Geometry: final body of the model. Coordinates: model frame, mm. Face numbers are marked on the shaded views. A direction names the side the tool comes from. Coordinates: 2 decimals unless noted, no trailing zeros. Write each loop counter-clockwise with the first axis right and the second up, starting at its lowest first coordinate (ties: lowest second). Pieces come first, ordered by that corner, then holes. Notation, with made-up numbers: (16.5, 84) - (45.5, 84) arc R24 cw to (45.5, 111) - close; hole circle Ø4 at (73.25, -14). An arc over 180 degrees is marked (long way). Put each result on its own line as item: value.
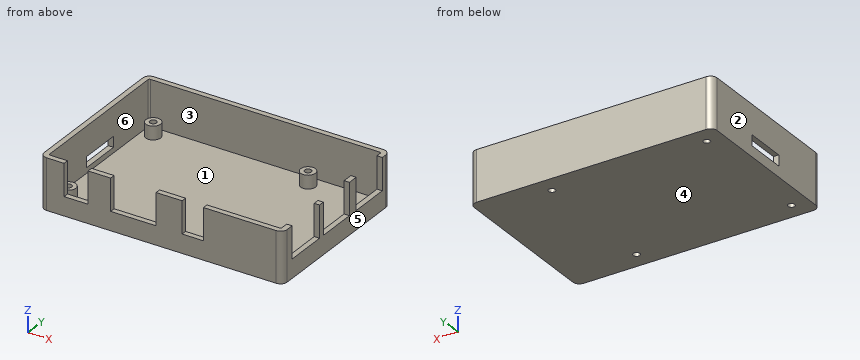
```python
from build123d import *

# Parameters (mm, degrees)
F0_W      = 87
F0_H      = 58
F1_DEPTH  = 2
F2_DEPTH  = 19
F3_R      = 2.75
F3_R_2    = 1.25
F4_DEPTH  = 5
F5_W      = 9
F5_H      = 2
F5_W_2    = 17
F5_W_3    = 8
F5_W_4    = 2
F5_H_2    = 15.9
F5_H_3    = 15.1
F6_DEPTH  = 12
F7_W      = 15.6
F7_H      = 4
F8_DEPTH  = 5
F9_R      = 0.5
F10_DEPTH = 2


with BuildPart() as f1:
    # F0 (on Top) → F1 (new body)
    with BuildSketch(Plane.XY):
        with BuildLine():
            ThreePointArc((0, 2.5), (0.732233047, 0.732233047), (2.5, 0))
            Line((2.5, 0), (88.5, 0))
            ThreePointArc((88.5, 0), (90.267766953, 0.732233047), (91, 2.5))
            Line((91, 2.5), (91, 59.5))
            ThreePointArc((91, 59.5), (90.267766953, 61.267766953), (88.5, 62))
            Line((88.5, 62), (2.5, 62))
            ThreePointArc((2.5, 62), (0.732233047, 61.267766953), (0, 59.5))
            Line((0, 59.5), (0, 2.5))
        make_face()
        with Locations((45.5, 31)):
            Rectangle(F0_W, F0_H, mode=Mode.SUBTRACT)
        with Locations((45.5, 31)):
            Rectangle(F0_W, F0_H)
    extrude(amount=F1_DEPTH)

    # F0 (on Top) → F2 (join)
    with BuildSketch(Plane.XY):
        with BuildLine():
            ThreePointArc((0, 2.5), (0.732233047, 0.732233047), (2.5, 0))
            Line((2.5, 0), (88.5, 0))
            ThreePointArc((88.5, 0), (90.267766953, 0.732233047), (91, 2.5))
            Line((91, 2.5), (91, 59.5))
            ThreePointArc((91, 59.5), (90.267766953, 61.267766953), (88.5, 62))
            Line((88.5, 62), (2.5, 62))
            ThreePointArc((2.5, 62), (0.732233047, 61.267766953), (0, 59.5))
            Line((0, 59.5), (0, 2.5))
        make_face()
        with Locations((45.5, 31)):
            Rectangle(F0_W, F0_H, mode=Mode.SUBTRACT)
    extrude(amount=F2_DEPTH)

    # F3 (on face) → F4 (join)
    with BuildSketch(Plane.XY.offset(2)):
        with Locations((6.5, 55.5)):
            Circle(F3_R)
        with Locations((6.5, 55.5)):
            Circle(F3_R_2, mode=Mode.SUBTRACT)
        with Locations((64.5, 6.5)):
            Circle(F3_R)
        with Locations((64.5, 6.5)):
            Circle(F3_R_2, mode=Mode.SUBTRACT)
        with Locations((6.5, 6.5)):
            Circle(F3_R)
        with Locations((6.5, 6.5)):
            Circle(F3_R_2, mode=Mode.SUBTRACT)
        with Locations((64.5, 55.5)):
            Circle(F3_R)
        with Locations((64.5, 55.5)):
            Circle(F3_R_2, mode=Mode.SUBTRACT)
    extrude(amount=F4_DEPTH)

    # F5 (on face) → F6 (cut)
    with BuildSketch(Plane.XY.offset(19)):
        with Locations((13.55, 1)):
            Rectangle(F5_W, F5_H)
        with Locations((35, 1)):
            Rectangle(F5_W_2, F5_H)
        with Locations((57.25, 1)):
            Rectangle(F5_W_3, F5_H)
        with Locations((90, 13.25)):
            Rectangle(F5_W_4, F5_H_2)
        with Locations((90, 30.95)):
            Rectangle(F5_W_4, F5_H_3)
        with Locations((90, 49.95)):
            Rectangle(F5_W_4, F5_H_3)
    extrude(amount=-F6_DEPTH, mode=Mode.SUBTRACT)

    # F7 (on face) → F8 (cut)
    with BuildSketch(Plane(origin=(0, 0, 0), x_dir=(0, -1, 0), z_dir=(-1, 0, 0))):
        with Locations((-31.7, 6)):
            Rectangle(F7_W, F7_H)
    extrude(amount=-F8_DEPTH, mode=Mode.SUBTRACT)

    # F9
    f9_edges = [f1.edges().sort_by_distance(p)[0] for p in [
        (2, 60, 10.5),
        (89, 60, 10.5),
        (2, 2, 10.5),
        (89, 2, 10.5),
    ]]
    fillet(f9_edges, radius=F9_R)

    # F10 (cut, through all): faces of the model
    f10_faces = [f1.faces().sort_by_distance(p)[0] for p in [
        (6.5, 55.5, 2),
        (64.5, 55.5, 2),
        (64.5, 6.5, 2),
        (6.5, 6.5, 2),
    ]]
    extrude(f10_faces, amount=-F10_DEPTH, mode=Mode.SUBTRACT)


solid = f1.part
```
1. Ray query, probe 1 along Y at (x, z) = (64.5, 1.6); probe 2 along X at (y, z) = (20, 6); probe 3 along Y at (x, z) = (48, 6.25). Return the intervals inside material, ascending. Write a range as from..to.
Answer below:
probe 1: y = 0..5.25, 7.75..54.25, 56.75..62
probe 2: x = 0..2, 89..91
probe 3: y = 0..2, 60..62
2. Section query C-C (x = 6.5). Return loops of the section in (y, z).
Answer below:
outline: (0, 0) - (5.25, 0) - (5.25, 7) - (3.75, 7) - (3.75, 2) - (2, 2) - (2, 19) - (0, 19) - close; (7.75, 0) - (54.25, 0) - (54.25, 7) - (52.75, 7) - (52.75, 2) - (9.25, 2) - (9.25, 7) - (7.75, 7) - close; (56.75, 0) - (62, 0) - (62, 19) - (60, 19) - (60, 2) - (58.25, 2) - (58.25, 7) - (56.75, 7) - close
3. Pin query (flat end, axial travel): pin 1 Ø1 at (x, z) = (90, 13.5) entering from +Y; pin 2 Ø8 at (x, y) = (61.5, 37.5) entering from +Z; pin 3 Ø2 at (x, y) = (64.5, 6.5) entering from +Z; pin 4 Ø0.6 at (y, z) = (0.5, 14.5) entering from -X. Return the tip coordinate at first contact, or that it passes through.
Answer below:
pin 1: stops at y = 61.79
pin 2: stops at z = 2
pin 3: passes through
pin 4: stops at x = 0.67
4. Section query A-A (z = 5). Count the separate pieces of the cut face and the enclosed holes in it, then the cut area to 3 significant figures.
Answer below:
separate pieces: 5
enclosed holes: 4
area: 635 mm²
5. Section query D-D (x = 71.5). Return loops of the section in (y, z).
Answer below:
outline: (0, 0) - (62, 0) - (62, 19) - (60, 19) - (60, 2) - (2, 2) - (2, 19) - (0, 19) - close
6. Mould query, pull axis X, two halves, no side actions, for the marked faces 1, 2, 3 and 4. Classes: +X half, -X half, draft (parallel to the pull), parting line (faces both ways), or undercut.
Answer below:
face 1: undercut
face 2: -X half
face 3: undercut
face 4: draft
7. Section query B-B (y = 55.5). Return loops of the section in (x, z).
Answer below:
outline: (0, 0) - (5.25, 0) - (5.25, 7) - (3.75, 7) - (3.75, 2) - (2, 2) - (2, 19) - (0, 19) - close; (7.75, 0) - (63.25, 0) - (63.25, 7) - (61.75, 7) - (61.75, 2) - (9.25, 2) - (9.25, 7) - (7.75, 7) - close; (65.75, 0) - (91, 0) - (91, 7) - (89, 7) - (89, 2) - (67.25, 2) - (67.25, 7) - (65.75, 7) - close
8. Set-up query: the marked faces 5 and 6. Return all of +Z, -Z, +X, -X, +Y, -Y with unobstructed straight access to the full face (end or side cutting, diameter ignored); none if empty.
Answer below:
face 5: +Z, -Z, +X, +Y, -Y
face 6: +Z
